```python
from build123d import *

# Parameters (mm, degrees)
F0_R     = 5.85
F0_R_2   = 3.75
F1_DEPTH = 170
F3_DEPTH = 45.001
F4_R     = 4.5
F5_DEPTH = 120.209153


with BuildPart() as f1:
    # F0 (on Front) → F1 (new body)
    with BuildSketch(Plane.XZ):
        with BuildLine():
            ThreePointArc((22.5, 20.5), (21.914214, 21.914214), (20.5, 22.5))
            Line((20.5, 22.5), (4.25, 22.5))
            Line((4.25, 22.5), (4.25, 18))
            Line((4.25, 18), (7, 18))
            Line((7, 18), (7, 9))
            Line((7, 9), (5, 7))
            Line((5, 7), (-5, 7))
            Line((-5, 7), (-7, 9))
            Line((-7, 9), (-7, 18))
            Line((-7, 18), (-4.25, 18))
            Line((-4.25, 18), (-4.25, 22.5))
            Line((-4.25, 22.5), (-20.5, 22.5))
            ThreePointArc((-20.5, 22.5), (-21.914214, 21.914214), (-22.5, 20.5))
            Line((-22.5, 20.5), (-22.5, 4.25))
            Line((-22.5, 4.25), (-18, 4.25))
            Line((-18, 4.25), (-18, 7))
            Line((-18, 7), (-9, 7))
            Line((-9, 7), (-7, 5))
            Line((-7, 5), (-7, -5))
            Line((-7, -5), (-9, -7))
            Line((-9, -7), (-18, -7))
            Line((-18, -7), (-18, -4.25))
            Line((-18, -4.25), (-22.5, -4.25))
            Line((-22.5, -4.25), (-22.5, -20.5))
            ThreePointArc((-22.5, -20.5), (-21.914214, -21.914214), (-20.5, -22.5))
            Line((-20.5, -22.5), (-4.25, -22.5))
            Line((-4.25, -22.5), (-4.25, -18))
            Line((-4.25, -18), (-7, -18))
            Line((-7, -18), (-7, -9))
            Line((-7, -9), (-5, -7))
            Line((-5, -7), (5, -7))
            Line((5, -7), (7, -9))
            Line((7, -9), (7, -18))
            Line((7, -18), (4.25, -18))
            Line((4.25, -18), (4.25, -22.5))
            Line((4.25, -22.5), (20.5, -22.5))
            ThreePointArc((20.5, -22.5), (21.914214, -21.914214), (22.5, -20.5))
            Line((22.5, -20.5), (22.5, -4.25))
            Line((22.5, -4.25), (18, -4.25))
            Line((18, -4.25), (18, -7))
            Line((18, -7), (9, -7))
            Line((9, -7), (7, -5))
            Line((7, -5), (7, 5))
            Line((7, 5), (9, 7))
            Line((9, 7), (18, 7))
            Line((18, 7), (18, 4.25))
            Line((18, 4.25), (22.5, 4.25))
            Line((22.5, 4.25), (22.5, 20.5))
        make_face()
        with Locations((-15, -15)):
            Circle(F0_R, mode=Mode.SUBTRACT)
        with Locations((15, -15)):
            Circle(F0_R, mode=Mode.SUBTRACT)
        with Locations((-15, 15)):
            Circle(F0_R, mode=Mode.SUBTRACT)
        Circle(F0_R_2, mode=Mode.SUBTRACT)
        with Locations((15, 15)):
            Circle(F0_R, mode=Mode.SUBTRACT)
    extrude(amount=F1_DEPTH)

    # F2 (on face) → F3 (cut, through all)
    with BuildSketch(Plane.YZ.offset(22.5)):
        Polygon((-170, 22.5), (-170, -22.5), (-125, 22.5), align=None)
        Polygon((0, -22.5), (0, 22.5), (-45, 22.5), align=None)
    extrude(amount=-F3_DEPTH, mode=Mode.SUBTRACT)

    # F4 (on face) → F5 (cut, through all)
    with BuildSketch(Plane(origin=(0, -11.25, -11.25), x_dir=(-1, 0, 0), z_dir=(0, 0.707107, 0.707107))):
        with Locations((0, 25.229708)):
            Circle(F4_R)
    extrude(amount=-F5_DEPTH, mode=Mode.SUBTRACT)


solid = f1.part
```
The listing builds one solid part. Answer for the finished solid, in the listing's coordinates (mm). A direction names the side the tool comes from. Round coordinates to 2 decimals unless told otherwise and drop trailing zeros. Loops run counter-clockwise (first coordinate to the right, second up) from the corner with the lowest first, then second, coordinate; pieces in that order, holes last.
Q1. For a pull along X with two mould halves and no side action, classify faces 5 (the face through (18, -84, 6)), 6 (the face through (-22.5, -84, 12)), 7 (the face through (-20, -84, 4.25)) as released by +X, released by -X, zero draft, split by the parting line, or undercut.
Q2. Section C-C, the plane y = -114 is taken. Count the separate pieces of the cut face and the enclosed holes in it, then the cut area to 3 significant figures.
Q3. Given pin 1 Ø5 at (x, z) = (8.5, 13) entering from -Y; pin 2 Ø5 at (y, z) = (-94.5, 1) entering from +X; pin 3 Ø3 at (y, z) = (-53, -2) entering from -X; pin 4 Ø4 at (x, z) = (4, 14.5) entering from +Y, each flat-ended and moving along its own axis, determine where each tip first touches the part or whether it passes through.
Q4. Which of the six approach directions +Z, -Z, +X, -X, +Y, -Y give full straight-line access (tool end or side, diameter ignored) to faces 1 (the face through (20, -84, 4.25)), 2 (the face through (-4.25, -84, 20)), 3 (the face through (4.25, -28, -20)), 4 (the face through (-18, -84, 6))?
Q5. Section B-B, the plane z = -15 is taken. Determine the outline of the cut face in (x, y).
Q6. Section A-A, the plane x = -15 is taken. Determine the outline of the cut face in (y, z).
Q7. Find the intervals of material crossed by line 1 (X direction, y = -57.5, z = -15); line 2 (Z direction, x = 15, y = -128), in increasing order.
Completed:
1. face 5: undercut
1. face 6: released by -X
1. face 7: zero draft
2. separate pieces: 1
2. enclosed holes: 5
2. area: 794 mm2
3. pin 1: stops at y = -137
3. pin 2: stops at x = 7
3. pin 3: stops at x = -7
3. pin 4: passes through
4. face 1: +X, +Y, -Y
4. face 2: +Z, +Y, -Y
4. face 3: -Z, +Y, -Y
4. face 4: +Y, -Y
5. outline: (-22.5, -162.5) - (-20.85, -162.5) - (-20.85, -7.5) - (-22.5, -7.5) - close; (-9.15, -162.5) - (-7, -162.5) - (-7, -7.5) - (-9.15, -7.5) - close; (7, -162.5) - (9.15, -162.5) - (9.15, -7.5) - (7, -7.5) - close; (20.85, -162.5) - (22.5, -162.5) - (22.5, -7.5) - (20.85, -7.5) - close
6. outline: (-170, -22.5) - (0, -22.5) - (-1.65, -20.85) - (-168.35, -20.85) - close; (-156.65, -9.15) - (-13.35, -9.15) - (-15.5, -7) - (-154.5, -7) - close; (-140.5, 7) - (-29.5, 7) - (-31.65, 9.15) - (-138.35, 9.15) - close; (-126.65, 20.85) - (-43.35, 20.85) - (-45, 22.5) - (-125, 22.5) - close
7. line 1: x = -22.5 to -20.85, -9.15 to -7, 7 to 9.15, 20.85 to 22.5
7. line 2: z = -22.5 to -20.85, -9.15 to -7, 7 to 9.15
